Geometry: final body of the model. Coordinates: model frame, mm. Give positions to 0.01 mm unless a question says otherwise; leave off trailing zeros. Write each loop counter-clockwise with the first axis right and the second up, starting at its lowest first coordinate (ties: lowest second). Pieces come first, ordered by that corner, then holes.
Q1. Pin query (flat end, axial travel): pin 1 Ø4 at (x, y) = (13.5, -3.5) entering from +Z; pin 2 Ø4 at (x, y) = (-0.5, -3) entering from -Z. Return the tip coordinate at first contact, or that it passes through.
Q2. Section C-C (y = 4). Return the cut outline in (x, z) (1 decimal), plus the area to 3 significant figures.
Q3. Section D-D (x = -152.4). Return the cut outline in (y, z) (3 decimals).
Q4. Line query: line 1 (X direction, y = 4.25, z = 228.5) (3 decimals); line 2 (X direction, y = 2, z = 136); line 3 (Z direction, x = 86, y = -4.25). Output: solid intervals per line, ascending.
Q5. Section B-B (z = -171.5). Return the cut outline in (x, y), plus the area to 3 significant figures.
Q6. Section A-A (z = -88.9). Return the cut outline in (x, y) (3 decimals), plus the area to 3 significant figures.
from build123d import *

# Parameters (mm, degrees)
F1_DEPTH = 6.35


with BuildPart() as f1:
    # F0 (on Front) → F1 (new body, symmetric)
    with BuildSketch(Plane.XZ):
        with BuildLine():
            Line((-165.735, 254), (-203.2, 254))
            Line((-203.2, 254), (-203.2, -44.172675))
            Line((-203.2, -44.172675), (-145.7325, -77.351551))
            ThreePointArc((-145.7325, -77.351551), (-140.851551, -95.5675), (-159.0675, -100.448449))
            Line((-159.0675, -100.448449), (-203.2, -74.968538))
            Line((-203.2, -74.968538), (-203.2, -254))
            Line((-203.2, -254), (-184.404, -254))
            Line((-184.404, -254), (-171.196, -254))
            Line((-171.196, -254), (-170.47146, -254))
            Line((-170.47146, -254), (-6.604, -254))
            Line((-6.604, -254), (-6.604, -12.7))
            Line((-6.604, -12.7), (6.604, -12.7))
            Line((6.604, -12.7), (6.604, -254))
            Line((6.604, -254), (171.196, -254))
            Line((171.196, -254), (184.404, -254))
            Line((184.404, -254), (188.53423, -254))
            Line((188.53423, -254), (203.2, -254))
            Line((203.2, -254), (203.2, -74.968538))
            Line((203.2, -74.968538), (159.0675, -100.448449))
            ThreePointArc((159.0675, -100.448449), (140.851551, -95.5675), (145.7325, -77.351551))
            Line((145.7325, -77.351551), (203.2, -44.172675))
            Line((203.2, -44.172675), (203.2, 254))
            Line((203.2, 254), (165.735, 254))
            Line((165.735, 254), (165.735, 215.9))
            ThreePointArc((165.735, 215.9), (152.4, 202.565), (139.065, 215.9))
            Line((139.065, 215.9), (139.065, 254))
            Line((139.065, 254), (101.6, 254))
            Line((101.6, 254), (101.6, 101.6))
            Line((101.6, 101.6), (0, 101.6))
            Line((0, 101.6), (-101.6, 101.6))
            Line((-101.6, 101.6), (-101.6, 254))
            Line((-101.6, 254), (-139.065, 254))
            Line((-139.065, 254), (-139.065, 215.9))
            ThreePointArc((-139.065, 215.9), (-152.4, 202.565), (-165.735, 215.9))
            Line((-165.735, 215.9), (-165.735, 254))
        make_face()
    extrude(amount=F1_DEPTH, both=True)


solid = f1.part
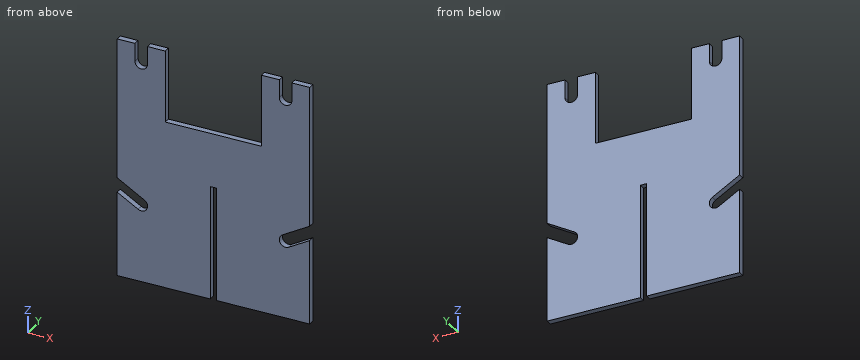
Computed:
1. pin 1: stops at z = 101.6
1. pin 2: stops at z = -12.7
2. outline: (-203.2, -254) - (-6.6, -254) - (-6.6, -12.7) - (6.6, -12.7) - (6.6, -254) - (203.2, -254) - (203.2, -75) - (159.1, -100.4) arc R13.3 cw to (145.7, -77.4) - (203.2, -44.2) - (203.2, 254) - (165.7, 254) - (165.7, 215.9) arc R13.3 cw to (139.1, 215.9) - (139.1, 254) - (101.6, 254) - (101.6, 101.6) - (-101.6, 101.6) - (-101.6, 254) - (-139.1, 254) - (-139.1, 215.9) arc R13.3 cw to (-165.7, 215.9) - (-165.7, 254) - (-203.2, 254) - (-203.2, -44.2) - (-145.7, -77.4) arc R13.3 cw to (-159.1, -100.4) - (-203.2, -75) - close
2. area: 166,000 mm2
3. outline: (-6.35, -254) - (6.35, -254) - (6.35, -102.235) - (-6.35, -102.235) - close; (-6.35, -73.502) - (6.35, -73.502) - (6.35, 202.565) - (-6.35, 202.565) - close
4. line 1: x = -203.2 to -165.735, -139.065 to -101.6, 101.6 to 139.065, 165.735 to 203.2
4. line 2: x = -203.2 to -101.6, 101.6 to 203.2
4. line 3: z = -254 to 101.6
5. outline: (-203.2, -6.35) - (-6.6, -6.35) - (-6.6, 6.35) - (-203.2, 6.35) - close; (6.6, -6.35) - (203.2, -6.35) - (203.2, 6.35) - (6.6, 6.35) - close
5. area: 4,990 mm2
6. outline: (-203.2, -6.35) - (-179.07, -6.35) - (-179.07, 6.35) - (-203.2, 6.35) - close; (-139.065, -6.35) - (-6.604, -6.35) - (-6.604, 6.35) - (-139.065, 6.35) - close; (6.604, -6.35) - (139.065, -6.35) - (139.065, 6.35) - (6.604, 6.35) - close; (179.07, -6.35) - (203.2, -6.35) - (203.2, 6.35) - (179.07, 6.35) - close
6. area: 3,980 mm2
